Build history of the part. All positions in model axes, mm. Coordinates: 2 decimals unless noted, no trailing zeros. Order: outer loops, then holes, each group sorted by start corner. A loop starts at its lowest first (then second) coordinate and runs counter-clockwise, first axis right, second up. Notation, with made-up numbers: (42.25, -11) - (58.25, -11) arc R25 cw to (58.25, 20) - close; hole circle Ø4 at (36.25, 80.25). An arc over 180 degrees is marked (long way). One line per item, written item: value.
from build123d import *

# Parameters (mm, degrees)
SKETCH3_R                            = 9.525
SKETCH3_R_2                          = 6.985
BOSS_EXTRUDE1_DEPTH                  = 7.9375
BOSS_EXTRUDE1_2_DEPTH                = 7.9375
BOSS_EXTRUDE2_REACH                  = 126.444
BOSS_EXTRUDE2_END_RADIUS             = 9.525
SKETCH4_R                            = 6.35
BOSS_EXTRUDE2_DIRECTION_2_REACH      = 126.444
BOSS_EXTRUDE2_DIRECTION_2_END_RADIUS = 9.525


with BuildPart() as part:
    # Sketch3 → Boss-Extrude1 (new, symmetric)
    with BuildSketch(Plane.XY):
        with Locations((-114.3, 0)):
            Circle(SKETCH3_R)
        with Locations((-114.3, 0)):
            Circle(SKETCH3_R_2, mode=Mode.SUBTRACT)
    extrude(amount=BOSS_EXTRUDE1_DEPTH, both=True)



with BuildPart() as body_2:
    # Sketch3 → Boss-Extrude1 2 (new, symmetric)
    with BuildSketch(Plane.XY):
        with Locations(Location((114.3, 0, 0), (0, 0, 180))):
            Circle(SKETCH3_R)
        with Locations(Location((114.3, 0, 0), (0, 0, 180))):
            Circle(SKETCH3_R_2, mode=Mode.SUBTRACT)
    extrude(amount=BOSS_EXTRUDE1_2_DEPTH, both=True)


with BuildPart() as part_1:
    add(part.part)

    add(body_2.part)  # Boss-Extrude2 merges body 2
    # Boss-Extrude2: up to this cylinder (the profile starts outside it)
    boss_extrude2_end = Plane(origin=(-114.3, 0, 0), z_dir=(0, 0, -1)) * Cylinder(BOSS_EXTRUDE2_END_RADIUS, 272.938, mode=Mode.PRIVATE)
    # Sketch4 → Boss-Extrude2 (add, up to the surface)
    with BuildSketch(Plane(origin=(0, 0, 0), x_dir=(0, 0, -1), z_dir=(1, 0, 0)), mode=Mode.PRIVATE) as boss_extrude2_sk1:
        with Locations(Location((0, 0, 0), (0, 0, 179.999999999))):
            Circle(SKETCH4_R)
    boss_extrude2_tool1 = extrude(boss_extrude2_sk1.sketch, amount=-BOSS_EXTRUDE2_REACH, mode=Mode.PRIVATE) - boss_extrude2_end
    add(boss_extrude2_tool1.solids().sort_by_distance((0, 0, 0))[0])

    # Boss-Extrude2 direction 2: up to this cylinder (the profile starts outside it)
    boss_extrude2_direction_2_end = Plane(origin=(114.3, 0, 0), z_dir=(0, 0, -1)) * Cylinder(BOSS_EXTRUDE2_DIRECTION_2_END_RADIUS, 272.938, mode=Mode.PRIVATE)
    # Sketch4 → Boss-Extrude2 direction 2 (add, up to the surface)
    with BuildSketch(Plane(origin=(0, 0, 0), x_dir=(0, 0, -1), z_dir=(1, 0, 0)), mode=Mode.PRIVATE) as boss_extrude2_direction_2_sk1:
        with Locations(Location((0, 0, 0), (0, 0, 179.999999999))):
            Circle(SKETCH4_R)
    boss_extrude2_direction_2_tool1 = extrude(boss_extrude2_direction_2_sk1.sketch, amount=BOSS_EXTRUDE2_DIRECTION_2_REACH, mode=Mode.PRIVATE) - boss_extrude2_direction_2_end
    add(boss_extrude2_direction_2_tool1.solids().sort_by_distance((0, 0, 0))[0])


solid = part_1.part
1. Band-saw the part on A-A, the plane x = -114.3. Give the cut face in (y, z) (1 decimal).
Values found:
outline: (-9.5, -7.9) - (-7, -7.9) - (-7, 7.9) - (-9.5, 7.9) - close; (7, -7.9) - (9.5, -7.9) - (9.5, 7.9) - (7, 7.9) - close
2. Band-saw the part on D-D, the plane x = -33. Give the cut face in (y, z), and give its area (3 significant figures).
Values found:
outline: circle Ø12.7 at (0, 0)
area: 127 mm2
3. Flat gauge pins, fed straight in: P1, Ø11, axis at x = -114.3, y = 0, coming from the -Z side; P2, Ø1.5, axis at x = -42, y = -2.5, coming from the +Z side; P3, Ø10, axis at x = 2, y = 5.5, coming from the -Z side; P4, Ø5, axis at y = -3, z = -3.5, coming from the +X side. Where does each tip first touch, or does it go through?
Values found:
P1: passes through
P2: stops at z = 6.1
P3: stops at z = -6.33
P4: stops at x = 123.81
4. Band-saw the part on B-B, the plane y = 0. Count the separate pieces of the cut face and the enclosed holes in it, and give its area (3 significant figures).
Values found:
separate pieces: 3
enclosed holes: 0
area: 2,820 mm2
5. Band-saw the part on C-C, the plane z = 0. Give the cut face in (x, y) (3 decimals).
Values found:
outline: (-107.2, -6.35) - (107.2, -6.35) arc R9.525 ccw (long way) to (107.2, 6.35) - (-107.2, 6.35) arc R9.525 ccw (long way) to start; hole circle Ø13.97 at (-114.3, 0); hole circle Ø13.97 at (114.3, 0)
6. Two-plate mould, pull along X, no slides. Class faces 1 (the face through (115.1, -7.1, -7.938)), 2 (the face through (123.816, -0.419, 0.111)), 3 (the face through (-1.5, -1.907, 6.057)): pulls with the +X half, pulls with the -X half, needs draft (parallel to the pull), parting line crosses it, or undercut.
Values found:
face 1: needs draft
face 2: undercut
face 3: undercut
7. Probe line 1 along X through (y, z) = (-0.5, 1.5); line 2 along X through (y, z) = (-6, 3.5); line 3 along X through (y, z) = (5, -3). List the from-to ranges inside material, lowest first.
Values found:
line 1: x = -123.81 to -121.27, -107.33 to 107.33, 121.27 to 123.81
line 2: x = -121.7 to -117.88, -110.72 to -106.9, 106.9 to 110.72, 117.88 to 121.7
line 3: x = -122.41 to -119.18, -109.42 to 109.42, 119.18 to 122.41
